from build123d import *

# Parameters (mm, degrees)
F1_DEPTH  = 21
F2_R      = 2
F3_DEPTH  = 50
F4_R      = 4.5
F5_DEPTH  = 4
F6_R      = 4.5
F7_DEPTH  = 4
F8_R      = 2
F9_DEPTH  = 15
F11_DEPTH = 12
F12_W     = 82.7163627307
F12_H     = 105.0548920631
F12_W_2   = 93.7405878742
F12_H_2   = 84.4749022052
F13_DEPTH = 25
F15_DEPTH = 50
F16_W     = 1
F16_H     = 20
F17_DEPTH = 65
F18_DEPTH = 25
F19_W     = 35
F19_H     = 35
F19_W_2   = 25
F19_H_2   = 25
F20_DEPTH = 10
F21_DEPTH = 25
F22_W     = 5
F22_H     = 8
F23_DEPTH = 41
F24_R     = 1
F25_R     = 2.75
F26_DEPTH = 25
F27_R     = 2


with BuildPart() as f1:
    # F0 (on Front) → F1 (new body)
    with BuildSketch(Plane.XZ):
        with BuildLine():
            ThreePointArc((44.6194845136, -22.563279942), (39.5277888838, -30.6195020528), (33, -37.563279942))
            Line((33, -37.563279942), (33, -79))
            Line((33, -79), (18.9958492358, -99))
            Line((18.9958492358, -99), (0, -99))
            Line((0, -99), (-33, -99))
            Line((-33, -99), (-33, -37.563279942))
            ThreePointArc((-33, -37.563279942), (-39.5277888838, -30.6195020528), (-44.6194845136, -22.563279942))
            Line((-44.6194845136, -22.563279942), (-50, -22.563279942))
            Line((-50, -22.563279942), (-50, -133))
            Line((-50, -133), (-33, -150))
            Line((-33, -150), (-33, -180))
            Line((-33, -180), (-33, -197))
            Line((-33, -197), (0, -197))
            Line((0, -197), (33, -197))
            Line((33, -197), (33, -180))
            Line((33, -180), (33, -150))
            Line((33, -150), (50, -133))
            Line((50, -133), (50, -22.563279942))
            Line((50, -22.563279942), (44.6194845136, -22.563279942))
        make_face()
    extrude(amount=F1_DEPTH)

    # F2 (on Right) → F3 (cut, symmetric)
    with BuildSketch(Plane.YZ):
        with Locations((-10.5, -55.10355)):
            Circle(F2_R)
        with Locations((-10.5, -85.60355)):
            Circle(F2_R)
    extrude(amount=F3_DEPTH, both=True, mode=Mode.SUBTRACT)

    # F4 (on face) → F5 (cut)
    with BuildSketch(Plane(origin=(-50, 0, 0), x_dir=(0, -1, 0), z_dir=(-1, 0, 0))):
        with Locations((10.5, -55.10355)):
            Circle(F4_R)
        with Locations((10.5, -85.60355)):
            Circle(F4_R)
    extrude(amount=-F5_DEPTH, mode=Mode.SUBTRACT)

    # F6 (on face) → F7 (cut)
    with BuildSketch(Plane.YZ.offset(50)):
        with Locations((-10.5, -55.10355)):
            Circle(F6_R)
        with Locations((-10.5, -85.60355)):
            Circle(F6_R)
    extrude(amount=-F7_DEPTH, mode=Mode.SUBTRACT)

    # F8 (on face) → F9 (cut)
    with BuildSketch(Plane(origin=(0, 0, -197), x_dir=(1, 0, 0), z_dir=(0, 0, -1))):
        with BuildLine():
            ThreePointArc((-23, 10.5), (-21, 8.5), (-19, 10.5))
            ThreePointArc((-19, 10.5), (-21, 12.5), (-23, 10.5))
        make_face()
        with Locations((21, 10.5)):
            Circle(F8_R)
    extrude(amount=-F9_DEPTH, mode=Mode.SUBTRACT)

    # F10 (on face) → F11 (cut)
    with BuildSketch(Plane.XZ.offset(21)):
        with BuildLine():
            ThreePointArc((0, -166.5), (-2, -168.5), (0, -170.5))
            Line((0, -170.5), (0, -166.5))
        make_face()
        with BuildLine():
            ThreePointArc((0, -131), (-2, -133), (0, -135))
            Line((0, -135), (0, -131))
        make_face()
        with BuildLine():
            Line((0, -131), (0, -135))
            ThreePointArc((0, -135), (1.4142135624, -134.4142135624), (2, -133))
            ThreePointArc((2, -133), (1.4142135624, -131.5857864376), (0, -131))
        make_face()
        with BuildLine():
            Line((0, -166.5), (0, -170.5))
            ThreePointArc((0, -170.5), (1.4142135624, -169.9142135624), (2, -168.5))
            ThreePointArc((2, -168.5), (1.4142135624, -167.0857864376), (0, -166.5))
        make_face()
    extrude(amount=-F11_DEPTH, mode=Mode.SUBTRACT)

    # F12 (on face) → F13 (cut)
    with BuildSketch(Plane.XZ.offset(21)):
        with Locations((60.3540306012, -151.5274460316)):
            Rectangle(F12_W, F12_H)
        with Locations((-27.8744447013, -151.5274460316)):
            Rectangle(F12_W_2, F12_H)
        with Locations((-27.8744447013, -56.7625488974)):
            Rectangle(F12_W_2, F12_H_2)
    extrude(amount=-F13_DEPTH, mode=Mode.SUBTRACT)

    # F14 (on face) → F15 (join)
    with BuildSketch(Plane(origin=(0, 0, 0), x_dir=(-1, 0, 0), z_dir=(0, 1, 0))):
        Polygon((-50, -79), (-50, -99), (24.0241140127, -99), (32, -99), (32, -79), (24.0241140127, -79), (-33, -79), align=None)
    extrude(amount=F15_DEPTH)

    # F16 (on face) → F17 (cut)
    with BuildSketch(Plane(origin=(-32, 0, 0), x_dir=(0, -1, 0), z_dir=(-1, 0, 0))):
        with Locations((-0.5, -89)):
            Rectangle(F16_W, F16_H)
    extrude(amount=-F17_DEPTH, mode=Mode.SUBTRACT)

    # F18 (add): a face of the model
    f18_faces = [f1.faces().sort_by_distance(p)[0] for p in [
        (28.3319497453, 0, -92.3333333333),
    ]]
    extrude(f18_faces, amount=F18_DEPTH)

    # F19 (on face) → F20 (join)
    with BuildSketch(Plane.XY.offset(-79)):
        with Locations((32.5, 32.5)):
            Rectangle(F19_W, F19_H)
        with Locations((32.5, 32.5)):
            Rectangle(F19_W_2, F19_H_2, mode=Mode.SUBTRACT)
    extrude(amount=F20_DEPTH)

    # F21 (cut): a face of the model
    f21_faces = [f1.faces().sort_by_distance(p)[0] for p in [
        (32.5, 32.5, -79),
    ]]
    extrude(f21_faces, amount=-F21_DEPTH, mode=Mode.SUBTRACT)

    # F22 (on face) → F23 (cut)
    with BuildSketch(Plane(origin=(0, 50, 0), x_dir=(-1, 0, 0), z_dir=(0, 1, 0))):
        with Locations((-32.5, -69)):
            Rectangle(F22_W, F22_H)
    extrude(amount=-F23_DEPTH, mode=Mode.SUBTRACT)

    # F24
    f24_edges = [f1.edges().sort_by_distance(p)[0] for p in [
        (35, 17.5, -73),
        (30, 17.5, -73),
        (35, 47.5, -73),
        (30, 47.5, -73),
    ]]
    fillet(f24_edges, radius=F24_R)

    # F25 (on face) → F26 (cut)
    with BuildSketch(Plane.XY.offset(-79)):
        with BuildLine():
            ThreePointArc((-17.5, 25.5), (-20.25, 28.25), (-23, 25.5))
            Line((-23, 25.5), (-17.5, 25.5))
        make_face()
        with BuildLine():
            Line((-17.5, 25.5), (-23, 25.5))
            ThreePointArc((-23, 25.5), (-20.25, 22.75), (-17.5, 25.5))
        make_face()
        with Locations((3.25, 25.5)):
            Circle(F25_R)
    extrude(amount=-F26_DEPTH, mode=Mode.SUBTRACT)

    # F27
    f27_edges = [f1.edges().sort_by_distance(p)[0] for p in [
        (50, -21, -60.78164),
        (50, 0, -50.78164),
        (50, 50, -84),
        (50, 15, -74),
        (15, 50, -74),
        (15, 15, -74),
        (-32, 50, -89),
        (-32, 1, -89),
    ]]
    fillet(f27_edges, radius=F27_R)


solid = f1.part
For this review, take the finished solid that the model builds, in its own axes (mm). A direction names the side the tool comes from. Give positions to 0.01 mm unless a question says otherwise; leave off trailing zeros. Loops run counter-clockwise (first coordinate to the right, second up) from the corner with the lowest first, then second, coordinate; pieces in that order, holes last.
Item 1: Take a section at C-C, the plane y = 36. State the section outline as (x, z) points, and give its area (3 significant figures).
Item 2: Take a section at A-A, the plane y = 25.5. State the section outline as (x, z) points.
Item 3: Draft analysis for pull direction Z (two halves, no side actions). For faces 5 (the flat face through (47, -10, -22.563)), 6 (the flat face through (46, -10, -88)), 7 (the flat face through (33, -10, -58)), state which applies: +Z half, -Z half, draft (parallel to the pull), parting line (faces both ways), or undercut.
Item 4: Insertion check: pin 1 (3.5 mm diameter, centred on y = 18.5, z = -70.5, fed in from -X); pin 2 (14.5 mm diameter, centred on y = -10.5, z = -55.1, fed in from -X); pin 3 (4.5 mm diameter, centred on y = -10.5, z = -55.1, fed in from +X). Each pin has a flat end and moves straight along its axis. Give the tip position at first contact, or say it passes through.
Item 5: Take a section at B-B, the plane x = 3.25. State the section outline as (y, z) points, and give its area (3 significant figures).
Item 6: Take a section at D-D, the plane z = -33. State the section outline as (x, y) points.
Item 7: Tool access review of faces 1 (the flat face through (33, 48, -73)), 2 (the flat face through (32, 20, -84)), 3 (the flat face through (32, 15, -74)), 4 (the flat face through (1, 1, -89)): name each direction out of +Z, -Z, +X, -X, +Y, -Y from which nothing blocks a thin tool from reaching the whole face with its end or side.
Item 8: For line 1 along Y through (x, z) = (27, -81); line 2 along X through (y, z) = (38, -73); line 3 along Z through (x, y) = (38.25, -10.5), list the stretches that pass through material, from the lowest coordinate up.
Calculated:
1. outline: (-32, -99) - (20, -99) - (20, -69) - (15, -69) - (15, -79) - (-32, -79) - close; (45, -99) - (50, -99) - (50, -69) - (45, -69) - close
1. area: 1,240 mm2
2. outline: (-32, -99) - (-23, -99) - (-23, -79) - (-32, -79) - close; (-17.5, -99) - (0.5, -99) - (0.5, -79) - (-17.5, -79) - close; (6, -99) - (20, -99) - (20, -69) - (15, -69) - (15, -79) - (6, -79) - close; (45, -99) - (50, -99) - (50, -69) - (45, -69) - close
3. face 5: +Z half
3. face 6: undercut
3. face 7: draft
4. pin 1: stops at x = 15
4. pin 2: stops at x = 33
4. pin 3: stops at x = 46
5. outline: (1, -99) - (22.75, -99) - (22.75, -79) - (1, -79) - close; (28.25, -99) - (50, -99) - (50, -79) - (28.25, -79) - close
5. area: 870 mm2
6. outline: (37.56, -21) - (48, -21) arc R2 ccw to (50, -19) - (50, -2) arc R2 ccw to (48, 0) - (37.56, 0) - close
7. face 1: +Z, +Y
7. face 2: +Z, -Z
7. face 3: +Z, +X, -X
7. face 4: +Z, -X, -Y
8. line 1: y = 1 to 20, 45 to 50
8. line 2: x = 15 to 20, 45 to 50
8. line 3: z = -99 to -87.6, -83.6 to -57.1, -53.1 to -32.2
